```python
from build123d import *

# Parameters (mm, degrees)
F0_W     = 125
F0_H     = 18
F1_DEPTH = 7.5
F2_W     = 16
F2_H     = 11
F3_DEPTH = 6
F4_R     = 2
F5_R     = 1


with BuildPart() as f1:
    # F0 (on Top) → F1 (new body)
    with BuildSketch(Plane.XY):
        with Locations((-2.4749040604, 16.1338936687)):
            Rectangle(F0_W, F0_H)
    extrude(amount=-F1_DEPTH)

    # F2 (on Top) → F3 (cut)
    with BuildSketch(Plane.XY):
        with Locations((-52.4749040604, 19.6338936687)):
            Rectangle(F2_W, F2_H)
        with Locations((-27.4749040604, 19.6338936687)):
            Rectangle(F2_W, F2_H)
        with Locations((-2.4749040604, 19.6338936687)):
            Rectangle(F2_W, F2_H)
        with Locations((22.5250959396, 19.6338936687)):
            Rectangle(F2_W, F2_H)
        with Locations((47.5250959396, 19.6338936687)):
            Rectangle(F2_W, F2_H)
    extrude(amount=-F3_DEPTH, mode=Mode.SUBTRACT)

    # F4
    f4_edges = [f1.edges().sort_by_distance(p)[0] for p in [
        (60.025096, 25.133894, -3.75),
        (60.025096, 7.133894, -3.75),
        (-64.974904, 25.133894, -3.75),
        (-64.974904, 7.133894, -3.75),
        (-2.474904, 7.133894, -7.5),
    ]]
    fillet(f4_edges, radius=F4_R)

    # F5
    f5_edges = [f1.edges().sort_by_distance(p)[0] for p in [
        (60.025096, 16.133894, 0),
        (59.43931, 7.71968, 0),
        (59.43931, 24.548107, 0),
        (-2.474904, 7.133894, 0),
        (56.775096, 25.133894, 0),
        (-64.389118, 7.71968, 0),
        (55.525096, 19.633894, 0),
        (-64.974904, 16.133894, 0),
        (47.525096, 14.133894, 0),
        (-64.389118, 24.548107, 0),
        (39.525096, 19.633894, 0),
        (-61.724904, 25.133894, 0),
        (35.025096, 25.133894, 0),
        (-60.474904, 19.633894, 0),
        (30.525096, 19.633894, 0),
        (-52.474904, 14.133894, 0),
        (22.525096, 14.133894, 0),
        (-44.474904, 19.633894, 0),
        (14.525096, 19.633894, 0),
        (-39.974904, 25.133894, 0),
        (10.025096, 25.133894, 0),
        (-35.474904, 19.633894, 0),
        (5.525096, 19.633894, 0),
        (-27.474904, 14.133894, 0),
        (-2.474904, 14.133894, 0),
        (-19.474904, 19.633894, 0),
        (-10.474904, 19.633894, 0),
        (-14.974904, 25.133894, 0),
    ]]
    fillet(f5_edges, radius=F5_R)


solid = f1.part
```
Could you check a few things on this model? Use its own coordinates, in mm. A direction names the side the tool comes from. Coordinates: 2 decimals unless noted, no trailing zeros. Order: outer loops, then holes, each group sorted by start corner. A loop starts at its lowest first (then second) coordinate and runs counter-clockwise, first axis right, second up. Notation, with made-up numbers: M 24,-27.5 L 64,-27.5 A37 cw 64,8.5 Z; hole C -13,79.5 d10. An arc over 180 degrees is marked long. Use a Markdown table: item, result. Add a question column.
Q1. If I drill on L1, parallel to X at y = 21.5, z = -2; L2, parallel to Z at x = 52, y = 16.5; L3, parallel to Y at x = -21, z = -1.5, over which ranges is the centre line in solid material (lowest first)?
Q2. I'm going to push flat-ended pins straight in: pin 1 (4 mm diameter, centred on x = -53, z = -2.5, fed in from +Y); pin 2 (9 mm diameter, centred on x = 26.5, y = 18.5, fed in from +Z); pin 3 (3.5 mm diameter, centred on x = -6, y = 21.5, fed in from +Z). Where does each tip first touch, or does it pass through?
Q3. Which directions (+Z, -Z, +X, -X, +Y, -Y) give clear straight access to the entire face, cutting with the end or side of a thin tool? Please do faces 1 (the flat face through (-3.3, 12.7, 0)), 2 (the flat face through (22, 20, -6)).
Q4. I want a section at A-A on x = 42. List the corners of the cut face in (y, z) for me.
Q5. We'd pull the mould along X, two halves only. Please class faces 3 (the flat face through (-10.475, 20, -3)), 4 (the flat face through (-3.3, 25.134, -6.4)), 5 (the cylindrical face through (59.424, 24.564, -4.296)): pulls with the +X half, pulls with the -X half, needs draft (parallel to the pull), parting line crosses it, or undercut.
Q6. I want a section at B-B on z = -4. List the corners of the cut face in (x, y) for me, then the cut area to 3 significant figures.
Checked values:
| question | item | result |
|---|---|---|
| 1 | L1 | -64.97 to -60.47, -44.47 to -35.47, -19.47 to -10.47, 5.53 to 14.53, 30.53 to 39.53, 55.53 to 60.03 |
| 1 | L2 | -7.5 to -6 |
| 1 | L3 | 7.13 to 14.13 |
| 2 | pin 1 | y = 14.13 |
| 2 | pin 2 | z = -0.15 |
| 2 | pin 3 | z = -6 |
| 3 | face 1 | +Z, +X, -X, +Y, -Y |
| 3 | face 2 | +Z, +Y |
| 4 | outline | M 7.13,-5.5 A2 ccw 9.13,-7.5 L 25.13,-7.5 L 25.13,-6 L 14.13,-6 L 14.13,-1 A1 ccw 13.13,0 L 8.13,0 A1 ccw 7.13,-1 Z |
| 5 | face 3 | undercut |
| 5 | face 4 | needs draft |
| 5 | face 5 | pulls with the +X half |
| 6 | outline | M -64.97,9.13 A2 ccw -62.97,7.13 L 58.03,7.13 A2 ccw 60.03,9.13 L 60.03,23.13 A2 ccw 58.03,25.13 L 55.53,25.13 L 55.53,14.13 L 39.53,14.13 L 39.53,25.13 L 30.53,25.13 L 30.53,14.13 L 14.53,14.13 L 14.53,25.13 L 5.53,25.13 L 5.53,14.13 L -10.47,14.13 L -10.47,25.13 L -19.47,25.13 L -19.47,14.13 L -35.47,14.13 L -35.47,25.13 L -44.47,25.13 L -44.47,14.13 L -60.47,14.13 L -60.47,25.13 L -62.97,25.13 A2 ccw -64.97,23.13 Z |
| 6 | area | 1,370 mm² |
